Geometry: see drawing. Coordinates: mm, zero at the bounding-box minimum. Coordinates: 2 decimals unless noted, no trailing zeros. Order: outer loops, then holes, each group sorted by start corner. A loop starts at its lowest first (then second) coordinate and runs counter-clockwise, first axis right, second up. Notation, with made-up numbers: M 53,69 L 94,69 A31 ccw 94,98 Z; hole C -0.5,75.25 d3. An arc over 180 degrees is marked long. Answer in a Markdown table with one row per item.
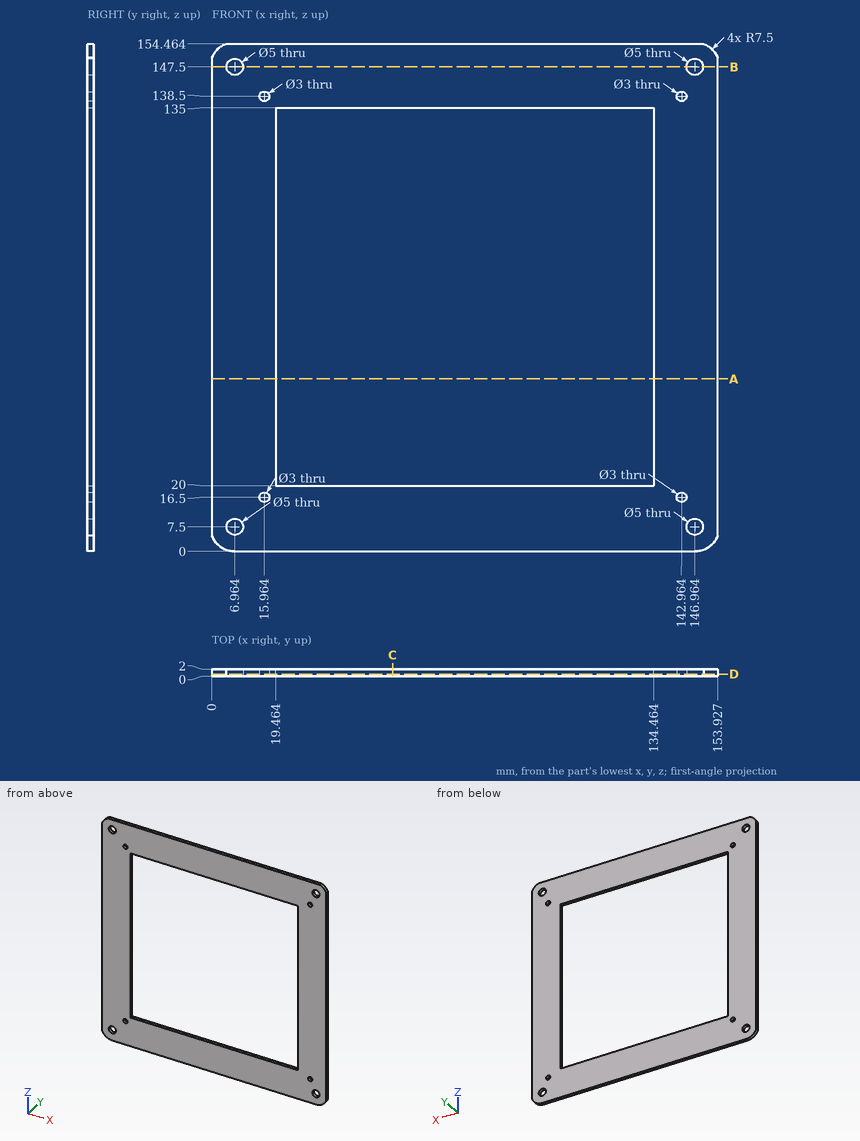
1) Cut plane B-B, the plane z = 147.5. Output: boundary loops of the cut face in (x, y).
Resolved:
| item | result |
|---|---|
| outline | M 0,0 L 4.46,0 L 4.46,2 L 0,2 Z; M 9.46,0 L 144.46,0 L 144.46,2 L 9.46,2 Z; M 149.46,0 L 153.93,0 L 153.93,2 L 149.46,2 Z |
2) Cut plane C-C, the plane x = 55. Output: boundary loops of the cut face in (y, z).
Resolved:
| item | result |
|---|---|
| outline | M 0,0 L 2,0 L 2,20 L 0,20 Z; M 0,135 L 2,135 L 2,154.46 L 0,154.46 Z |
3) Cut plane D-D, the plane y = 0.55. State how many separate pieces and enclosed holes the cut face has, and give its area (3 significant figures).
Resolved:
| item | result |
|---|---|
| separate pieces | 1 |
| enclosed holes | 9 |
| area | 10,400 mm2 |
4) Cut plane A-A, the plane z = 52.5. Output: boundary loops of the cut face in (x, y).
Resolved:
| item | result |
|---|---|
| outline | M 0,0 L 19.46,0 L 19.46,2 L 0,2 Z; M 134.46,0 L 153.93,0 L 153.93,2 L 134.46,2 Z |
5) Material intervals for probe 1 along X at (y, z) = (1.35, 16.5); probe 2 along X at (y, z) = (0.7, 7.5); probe 3 along X at (y, z) = (1, 49.5), sorted ascending.
Resolved:
| item | result |
|---|---|
| probe 1 | x = 0 to 14.46, 17.46 to 141.46, 144.46 to 153.93 |
| probe 2 | x = 0 to 4.46, 9.46 to 144.46, 149.46 to 153.93 |
| probe 3 | x = 0 to 19.46, 134.46 to 153.93 |
